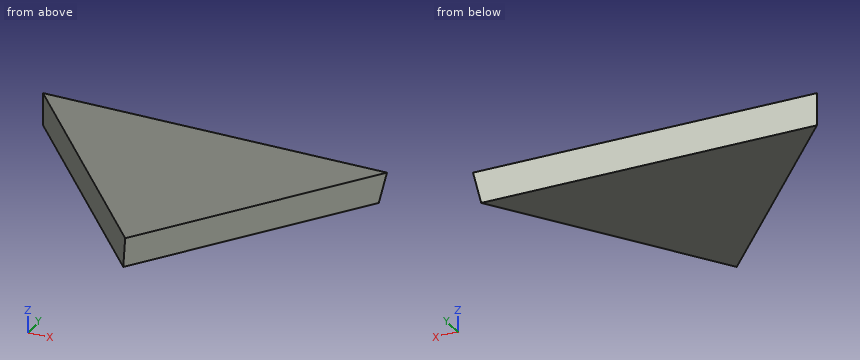
```python
from build123d import *

# Parameters (mm, degrees)
BOSS_EXTRUDE1_DEPTH = 70
CHAMFER1_SIZE2      = 4.18941816
CHAMFER1_SIZE       = 70
CHAMFER2_SIZE       = 7.017777763
CHAMFER2_SIZE_2     = 70


# Some blends are built 0.0001 mm under size
with BuildPart() as part:
    # Sketch1 → Boss-Extrude1 (new body)
    with BuildSketch(Plane(origin=(5.473822054, -457.937984789, -3307.31325441), x_dir=(-0.9856470342360776, 0.16521656475401902, -0.03469020946183102), z_dir=(-0.0017423663357502073, 0.19552071957465159, 0.980698023030822))):
        Polygon((1127.410622311, 6899.993028511), (1231.788289667, 7721.098906243), (1938.364522736, 7065.713670786), align=None)
    extrude(amount=-BOSS_EXTRUDE1_DEPTH)

    # Chamfer1
    chamfer1_edges = [part.edges().sort_by_distance(p)[0] for p in [
        (-2804.812562525, -7356.820333598, -2008.261086677),
    ]]
    chamfer1_side = [part.faces().sort_by_distance(p)[0] for p in [
        (-2804.812708515, -7356.803951237, -2008.178915595),
    ]]
    chamfer(chamfer1_edges, length=CHAMFER1_SIZE - 0.0001, length2=CHAMFER1_SIZE2 - 0.0001, reference=chamfer1_side[0])  # a hair under: the kernel refuses the full size

    # Chamfer2
    # the kernel refuses this chamfer: 70, 7.017777763 mm, written as the material it takes off along each edge
    with BuildSketch(Plane(origin=(-3274.435511319, -6987.276794808, -2082.770948142), x_dir=(0.030469156507814454, -0.9854547133895118, -0.1671844441331112), z_dir=(0.999487976226041, 0.031673079457915976, -0.004538878410539619))) as chamfer2_piece_1:
        Polygon((CHAMFER2_SIZE * 0.934223811245, -CHAMFER2_SIZE * 0.356687356966), (-CHAMFER2_SIZE_2 * 0.356687356946, -CHAMFER2_SIZE_2 * 0.93422381119), (0, 0), align=None)
    extrude(amount=1186.493835622, mode=Mode.SUBTRACT)
    with BuildSketch(Plane(origin=(-2217.332595505, -6784.751941859, -2121.270000408), x_dir=(0.0019280825655142314, 0.19442255260126845, 0.9809159767980269), z_dir=(-0.2917562783292002, -0.9381311781639606, 0.1865158615565802))) as chamfer2_piece_2:
        Polygon((CHAMFER2_SIZE_2 * 0.999992637165, CHAMFER2_SIZE_2 * 0.00383739696559), (-CHAMFER2_SIZE * 0.00383739696579, CHAMFER2_SIZE * 0.999992637223), (0, 0), align=None)
    extrude(amount=1186.493835622, mode=Mode.SUBTRACT)


solid = part.part
```
Verification items for the finished model (mm, model axes). Coordinates: 2 decimals unless noted, no trailing zeros. Loops run counter-clockwise (first coordinate to the right, second up) from the corner with the lowest first, then second, coordinate; pieces in that order, holes last. Notation, with made-up numbers: (-11.75, 44.25) - (17.25, 44.25) arc R29 cw to (17.25, 72.25) - close; hole circle Ø2 at (-15.75, 27.25). An arc over 180 degrees is marked (long way). Answer as a JSON object with one key per item and string values.
(1) Scan lines: line 1 along X through (y, z) = (-7358.5, -2002); line 2 along Z through (x, y) = (-2386.5, -7105); line 3 along Z through (x, y) = (-2361, -7056). Record each from-to range of solid material in increasing order.
Response:
{"line 1": "x = -2797.79 to -2402.89", "line 2": "z = -2057.72 to -1986.35", "line 3": "z = -2067.45 to -1996.07"}
(2) Cross-section at D-D, the plane x = -2486.5. Record the boundary of the cut face in (y, z).
Response:
{"outline": "(-7636.17, -1880.62) - (-7626.66, -1953.9) - (-6969.19, -2084.98) - (-6948.62, -2017.7) - close"}
(3) Go/stop test with flat-tipped pins: pin 1 Ø1 at (y, z) = (-7502, -1957) entering from +X; pin 2 Ø1.5 at (y, z) = (-7542.5, -1901.5) entering from +X; pin 3 Ø3 at (y, z) = (-7373, -1980.5) entering from -X. Record where each tip stops, or that it passes through.
Response:
{"pin 1": "stops at x = -2446.67", "pin 2": "stops at x = -2457.22", "pin 3": "stops at x = -2786.24"}
